```python
from build123d import *

# Parameters (mm, degrees)
BOSS_EXTRUDE1_DEPTH   = 2.85
BOSS_EXTRUDE2_DEPTH   = 2.9
F_2_0MM_DOWEL_HOLE1_D = 2


with BuildPart() as part:
    # Sketch1 → Boss-Extrude1 (new, symmetric)
    with BuildSketch(Plane(origin=(0, 0, 0), x_dir=(1, 0, 0), z_dir=(0, 1, 0))):
        Polygon((-6.4, 3.25), (-6.4, -0.75), (-1.25, -0.75), (-1.25, -2.25), (1.25, -2.25), (1.25, -0.75), (6.4, -0.75), (6.4, 3.25), align=None)
    extrude(amount=BOSS_EXTRUDE1_DEPTH, both=True)

    # Sketch1<3> → Boss-Extrude2 (add, symmetric)
    with BuildSketch(Plane(origin=(0, 0, 0), x_dir=(1, 0, 0), z_dir=(0, 1, 0))):
        Polygon((-1.25, -0.75), (-6.45, -0.75), (-6.45, -3.25), (-4.75, -3.25), (-4.25, -3.75), (-2.25, -3.75), (-1.75, -3.25), (1.75, -3.25), (2.25, -3.75), (4.25, -3.75), (4.75, -3.25), (6.45, -3.25), (6.45, -0.75), (1.25, -0.75), (1.25, -2.25), (-1.25, -2.25), align=None)
    extrude(amount=BOSS_EXTRUDE2_DEPTH, both=True)

    # Ø2.0mm Dowel Hole1 (through all)
    with Locations(Plane(origin=(0, -2.9, 0), x_dir=(-1, 0, 0), z_dir=(0, -1, 0))):
        with Locations((3.25, -2.05), (-3.25, -2.05)):
            Hole(F_2_0MM_DOWEL_HOLE1_D / 2)


solid = part.part
```
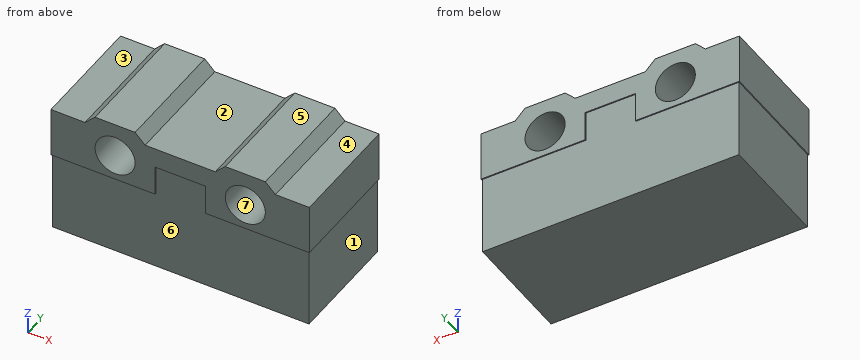
CAD build for the part. Positions are in the model's coordinates, mm. Face numbers are marked on the shaded views. A direction names the side the tool comes from. Round coordinates to 2 decimals unless told otherwise and drop trailing zeros. Order: outer loops, then holes, each group sorted by start corner. A loop starts at its lowest first (then second) coordinate and runs counter-clockwise, first axis right, second up. Notation, with made-up numbers: (55.5, 12.5) - (100.5, 12.5) arc R9 ccw to (100.5, 18.5) - close; hole circle Ø2 at (55, 81). An arc over 180 degrees is marked (long way). Use CSV: the item, a comma, the result in double quotes. Start each with the question number.
1) Pin check, flat tips, straight feed: pin 1 Ø2.5 at (x, z) = (-3.25, 2.05) entering from -Y; pin 2 Ø3 at (x, y) = (0.5, -1) entering from +Z; pin 3 Ø1.5 at (x, z) = (2.5, -0.5) entering from +Y; pin 4 Ø1.9 at (x, y) = (-6, -1) entering from +Z. Stop position of each tip, or through.
2) Wall check: L1, parallel to Z at x = -3.25, y = -0.55; L2, parallel to X at y = -2.2, z = -1.5; L3, parallel to X at y = 0.5, z = 1.5. Give the ranges that are in metal, low to high. Write a range as [from, to].
3) Saw through at B-B (y = 2.5). List the corners of the cut face in (x, z).
4) Tool access for the marked faces 1, 2, 3 and 4: list every direction of +Z, -Z, +X, -X, +Y, -Y with a clear straight run to the whole face (end or side of a thin tool).
5) Two-plate mould, pull along Z, no slides. Class the marked faces 5, 6 and 7: pulls with the +Z half, pulls with the -Z half, needs draft (parallel to the pull), parting line crosses it, or undercut.
6) Saw through at C-C (x = 3.25). List the corners of the cut face in (y, z), and give its area (3 significant figures).
7) Saw through at A-A (z = 2.05). List the corners of the cut face in (x, y), and give its area (3 significant figures).
8) Saw through at D-D (x = 1.5). List the corners of the cut face in (y, z), and give its area (3 significant figures).
Values follow:
1,pin 1,"stops at y = -2.9"
1,pin 2,"stops at z = 3.5"
1,pin 3,"stops at y = 2.85"
1,pin 4,"stops at z = 3.25"
2,L1,"z = [-3.25, 1.05], [3.05, 3.75]"
2,L2,"x = [-6.4, 6.4]"
2,L3,"x = [-6.45, -4.09], [-2.41, 2.41], [4.09, 6.45]"
3,outline,"(-6.45, 0.75) - (-6.4, 0.75) - (-6.4, -3.25) - (6.4, -3.25) - (6.4, 0.75) - (6.45, 0.75) - (6.45, 3.25) - (4.75, 3.25) - (4.25, 3.75) - (2.25, 3.75) - (1.75, 3.25) - (-1.75, 3.25) - (-2.25, 3.75) - (-4.25, 3.75) - (-4.75, 3.25) - (-6.45, 3.25) - close; hole circle Ø2 at (-3.25, 2.05); hole circle Ø2 at (3.25, 2.05)"
4,face 1,"-Z, +X, +Y, -Y"
4,face 2,"+Z, +Y, -Y"
4,face 3,"+Z, -X, +Y, -Y"
4,face 4,"+Z, +X, +Y, -Y"
5,face 5,"pulls with the +Z half"
5,face 6,"needs draft"
5,face 7,"undercut"
6,outline,"(-2.9, 0.75) - (-2.85, 0.75) - (-2.85, -3.25) - (2.85, -3.25) - (2.85, 0.75) - (2.9, 0.75) - (2.9, 1.05) - (-2.9, 1.05) - close; (-2.9, 3.05) - (2.9, 3.05) - (2.9, 3.75) - (-2.9, 3.75) - close"
6,area,"28.6 mm2"
7,outline,"(-6.45, -2.9) - (-4.25, -2.9) - (-4.25, 2.9) - (-6.45, 2.9) - close; (-2.25, -2.9) - (-1.25, -2.9) - (-1.25, -2.85) - (1.25, -2.85) - (1.25, -2.9) - (2.25, -2.9) - (2.25, 2.9) - (1.25, 2.9) - (1.25, 2.85) - (-1.25, 2.85) - (-1.25, 2.9) - (-2.25, 2.9) - close; (4.25, -2.9) - (6.45, -2.9) - (6.45, 2.9) - (4.25, 2.9) - close"
7,area,"51.4 mm2"
8,outline,"(-2.9, 0.75) - (-2.85, 0.75) - (-2.85, -3.25) - (2.85, -3.25) - (2.85, 0.75) - (2.9, 0.75) - (2.9, 3.25) - (-2.9, 3.25) - close"
8,area,"37.3 mm2"
